Build history of the part. All positions in model axes, mm. A direction names the side the tool comes from. Coordinates: 2 decimals unless noted, no trailing zeros. Write each loop counter-clockwise with the first axis right and the second up, starting at its lowest first coordinate (ties: lowest second). Pieces come first, ordered by that corner, then holes. Notation, with made-up numbers: (48, -23) -> (53, -23) arc R15 cw to (53, -17) -> close; hole circle Ø11 at (85, 8.25). An arc over 180 degrees is marked (long way). Write each question's results on one line, items separated by ' | '. Start each with the question number.
Q1. Two-plate mould, pull along Z, no slides. Class faces 1 (the face through (-15.8, 1.8, 3.9)), 2 (the face through (-11.3, -0.5, 0.925)), 3 (the face through (0, 1, -27.075)), 4 (the face through (-12.515, 0.301, 3.967)): released by +Z, released by -Z, zero draft, split by the parting line, or undercut.
Q2. Drop flat-ended pins along their axis: pin 1 Ø0.5 at (x, y) = (7, 3) entering from +Z; pin 2 Ø1.6 at (y, z) = (4, 4) entering from +X; pin 3 Ø0.8 at (x, z) = (5.5, -25.5) entering from +Y. Give the stop position or say it passes through.
Q3. Drill centre lines: line 1 (Z direction, x = -11, y = -0.75) (3 decimals); line 2 (Z direction, x = 11.5, y = 1.3) (3 decimals); line 3 (X direction, y = -0.35, z = 15). Where is each one in solid material? Low to high.
Q4. Saw through at C-C on y = 1.65. Give the cut face in (x, z) (3 decimals), and give its area (3 significant figures).
Q5. Saw through at A-A on x = 1. Give the cut face in (y, z) (3 decimals).
Q6. Saw through at B-B on z = 17. Give the cut face in (x, y).
Q7. Tool access for faces 5 (the face through (-14.3, -0.5, 19.2)), 6 (the face through (-1, 3.1, -25)), 7 (the face through (-11.3, -0.5, 7.925)), 8 (the face through (-13.31, 0.285, 1.624)): list every direction of +Z, -Z, +X, -X, +Y, -Y with a clear straight run to the whole face (end or side of a thin tool).
from build123d import *

# Parameters (mm, degrees)
SKETCH2_W           = 28.600197044
SKETCH2_H           = 54.15
BOSS_EXTRUDE1_DEPTH = 1
SKETCH2_3_W         = 28.600197044
SKETCH2_3_H         = 54.15
SKETCH2_3_W_2       = 25.600197044
SKETCH2_3_H_2       = 51.15
BOSS_EXTRUDE2_DEPTH = 3.1
SKETCH3_W           = 25.88588247
SKETCH3_H           = 51.15
CUT_EXTRUDE1_DEPTH  = 3.1
BOSS_EXTRUDE3_DEPTH = 4
SKETCH5_W           = 28.600197044
SKETCH5_H           = 2.5
BOSS_EXTRUDE4_DEPTH = 1
FILLET1_R           = 1
FILLET2_R           = 0.5
SKETCH7_W           = 6
SKETCH7_H           = 1
CUT_EXTRUDE2_DEPTH  = 1
FILLET3_R           = 0.5
FILLET4_R           = 0.5


with BuildPart() as part:
    # Sketch2 → Boss-Extrude1 (new body)
    with BuildSketch(Plane(origin=(0, 0, 0), x_dir=(1, 0, 0), z_dir=(0, 1, 0))):
        Rectangle(SKETCH2_W, SKETCH2_H)
    extrude(amount=-BOSS_EXTRUDE1_DEPTH)

    # Sketch2<3> → Boss-Extrude2 (add)
    with BuildSketch(Plane(origin=(0, 0, 0), x_dir=(1, 0, 0), z_dir=(0, 1, 0))):
        Rectangle(SKETCH2_3_W, SKETCH2_3_H)
        Rectangle(SKETCH2_3_W_2, SKETCH2_3_H_2, mode=Mode.SUBTRACT)
    extrude(amount=BOSS_EXTRUDE2_DEPTH)

    # Sketch3 → Cut-Extrude1 (cut)
    with BuildSketch(Plane(origin=(0, 3.1, 0), x_dir=(1, 0, 0), z_dir=(0, 1, 0))):
        with Locations((-6.642842713, 0)):
            Rectangle(SKETCH3_W, SKETCH3_H)
    extrude(amount=-CUT_EXTRUDE1_DEPTH, mode=Mode.SUBTRACT)

    # Sketch4 → Boss-Extrude3 (add)
    with BuildSketch(Plane.XY.offset(1.925)):
        Polygon((-14.300098522, 0), (-12.800098522, 0), (-12.800098522, 3.1), (-11.300098522, 3.1), (-11.300098522, 4.6), (-17.300098522, 4.6), (-14.300098522, -1), align=None)
    extrude(amount=BOSS_EXTRUDE3_DEPTH)

    # Sketch5 → Boss-Extrude4 (add)
    with BuildSketch(Plane(origin=(0, 3.1, 0), x_dir=(1, 0, 0), z_dir=(0, 1, 0))):
        with Locations((0, 25.825)):
            Rectangle(SKETCH5_W, SKETCH5_H)
    extrude(amount=BOSS_EXTRUDE4_DEPTH)

    # Fillet1
    fillet1_edges = [part.edges().sort_by_distance(p)[0] for p in [
        (-13.550098522, 0, 1.925),
        (-12.800098522, 0, 3.925),
        (-13.550098522, 0, 5.925),
    ]]
    fillet(fillet1_edges, radius=FILLET1_R)

    # Fillet2
    fillet2_edges = [part.edges().sort_by_distance(p)[0] for p in [
        (14.300098522, 3.1, 1.25),
        (0, 3.1, 27.075),
        (12.800098522, 3.1, 0.5),
        (-0.75, 3.1, 25.575),
        (-14.300098522, 4.1, -25.825),
        (0, 4.1, -24.575),
        (14.300098522, 4.1, -25.825),
        (0, 4.1, -27.075),
    ]]
    fillet(fillet2_edges, radius=FILLET2_R)

    # Sketch7 → Cut-Extrude2 (cut)
    with BuildSketch(Plane(origin=(0, 0, 0), x_dir=(1, 0, 0), z_dir=(0, 1, 0))):
        with Locations((-11.300098522, -0.425)):
            Rectangle(SKETCH7_W, SKETCH7_H)
        with Locations((-11.300098522, -7.425)):
            Rectangle(SKETCH7_W, SKETCH7_H)
    extrude(amount=-CUT_EXTRUDE2_DEPTH, mode=Mode.SUBTRACT)

    # Fillet3
    fillet3_edges = [part.edges().sort_by_distance(p)[0] for p in [
        (-14.300098522, -0.5, 0.925),
        (-14.300098522, -0.5, -0.075),
        (-8.300098522, -0.5, -0.075),
        (-8.300098522, -0.5, 0.925),
        (-14.300098522, -0.5, 7.925),
        (-14.300098522, -0.5, 6.925),
        (-8.300098522, -0.5, 6.925),
        (-8.300098522, -0.5, 7.925),
    ]]
    fillet(fillet3_edges, radius=FILLET3_R - 0.0001)  # a hair under: the kernel refuses the full size

    # Fillet4
    fillet4_edges = [part.edges().sort_by_distance(p)[0] for p in [
        (12.800098522, 0, 0),
        (-0.75, 0, -25.575),
        (-0.75, 0, 25.575),
    ]]
    fillet(fillet4_edges, radius=FILLET4_R)


solid = part.part
Returned:
1) face 1: zero draft | face 2: undercut | face 3: released by -Z | face 4: undercut
2) pin 1: stops at z = 27.05 | pin 2: stops at x = -11.3 | pin 3: stops at y = 4.1
3) line 1: z = -27.075 to -0.075, 0.925 to 6.925, 7.925 to 27.075 | line 2: z = -27.075 to -25.575, 25.575 to 27.075 | line 3: x = -14.3 to 14.3
4) outline: (-15.72, 1.925) -> (-12.8, 1.925) -> (-12.8, 5.925) -> (-15.72, 5.925) -> close; (-14.3, -27.075) -> (14.3, -27.075) -> (14.3, 27.075) -> (-14.3, 27.075) -> (-14.3, 25.575) -> (12.8, 25.575) -> (12.8, -25.575) -> (-14.3, -25.575) -> close | area: 174 mm2
5) outline: (-1, -27.075) -> (3.6, -27.075) arc R0.5 ccw to (4.1, -26.575) -> (4.1, -25.075) arc R0.5 ccw to (3.6, -24.575) -> (3.1, -24.575) -> (3.1, -25.575) -> (0.5, -25.575) arc R0.5 cw to (0, -25.075) -> (0, 25.075) arc R0.5 cw to (0.5, 25.575) -> (2.6, 25.575) arc R0.5 ccw to (3.1, 26.075) -> (3.1, 26.575) arc R0.5 ccw to (2.6, 27.075) -> (-1, 27.075) -> close
6) outline: (-14.3, -1) -> (14.3, -1) -> (14.3, 2.6) arc R0.5 ccw to (13.8, 3.1) -> (13.3, 3.1) arc R0.5 ccw to (12.8, 2.6) -> (12.8, 0.5) arc R0.5 cw to (12.3, 0) -> (-14.3, 0) -> close
7) face 5: +Z, -X, +Y, -Y | face 6: -X | face 7: -X, +Y, -Y | face 8: -X, +Y
